Here's how the part is built. I have some questions about the finished solid (model axes, mm). Face numbers are marked on the shaded views. A direction names the side the tool comes from. Round coordinates to 2 decimals unless told otherwise and drop trailing zeros. Loops run counter-clockwise (first coordinate to the right, second up) from the corner with the lowest first, then second, coordinate; pieces in that order, holes last. Notation, with made-up numbers: M 12.25,30.25 L 30.25,30.25 A27 cw 30.25,52.25 Z; hole C -4,69 d9. An arc over 180 degrees is marked long. Answer as a JSON object with one key per item and string values.
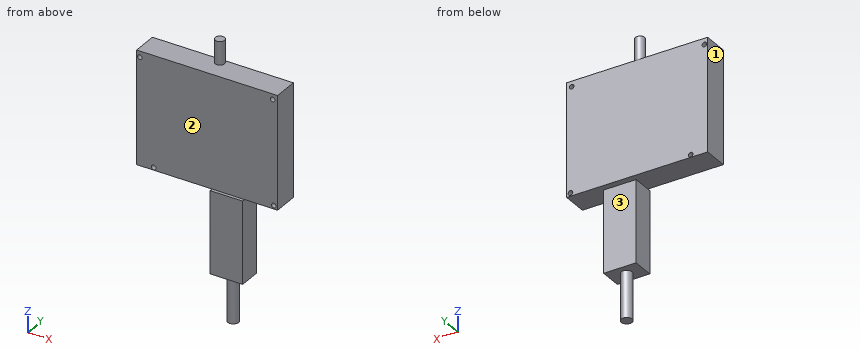
from build123d import *

# Parameters (mm, degrees)
SKETCH1_W                = 91.1
SKETCH1_H                = 73
SKETCH1_R                = 1.5
BOSS_EXTRUDE1_DEPTH      = 16.1
SKETCH2_R                = 3
BOSS_EXTRUDE2_DEPTH      = 15
BOSS_EXTRUDE3_DEPTH      = 12
BOSS_EXTRUDE3_DEPTH_BACK = 2
SKETCH3_W                = 21
SKETCH3_H                = 53
SKETCH4_R                = 3.5
BOSS_EXTRUDE4_DEPTH      = 30


with BuildPart() as part:
    # Sketch1 → Boss-Extrude1 (new body)
    with BuildSketch(Plane(origin=(0, 0, 0), x_dir=(1, 0, 0), z_dir=(0, 1, 0))):
        Rectangle(SKETCH1_W, SKETCH1_H)
        with Locations(Location((-34.59, 34.8, 0), (0, 0, 270))):
            Circle(SKETCH1_R, mode=Mode.SUBTRACT)
        with Locations(Location((43.1, 34.36, 0), (0, 0, 270))):
            Circle(SKETCH1_R, mode=Mode.SUBTRACT)
        with Locations(Location((42.3, -32.93, 0), (0, 0, 270))):
            Circle(SKETCH1_R, mode=Mode.SUBTRACT)
        with Locations(Location((-43.5, -32.58, 0), (0, 0, 270))):
            Circle(SKETCH1_R, mode=Mode.SUBTRACT)
    extrude(amount=BOSS_EXTRUDE1_DEPTH)

    # Sketch2 → Boss-Extrude2 (add)
    with BuildSketch(Plane.XY.offset(36.5)):
        with Locations(Location((0, 13.1, 0), (0, 0, 90))):
            Circle(SKETCH2_R)
    extrude(amount=BOSS_EXTRUDE2_DEPTH)

    # Sketch3 → Boss-Extrude3 (add, two sides: drawn at the far end of the back side and taken through both)
    with BuildSketch(Plane(origin=(0, 0, 0), x_dir=(1, 0, 0), z_dir=(0, 1, 0)).offset(-BOSS_EXTRUDE3_DEPTH_BACK)):
        with Locations((13.75, 63)):
            Rectangle(SKETCH3_W, SKETCH3_H)
    extrude(amount=BOSS_EXTRUDE3_DEPTH + BOSS_EXTRUDE3_DEPTH_BACK)

    # Sketch4 → Boss-Extrude4 (add)
    with BuildSketch(Plane(origin=(0, 0, -89.5), x_dir=(-1, 0, 0), z_dir=(0, 0, -1))):
        with Locations((-13.75, 5)):
            Circle(SKETCH4_R)
    extrude(amount=BOSS_EXTRUDE4_DEPTH)


solid = part.part
Item 1: For P1, Ø8, axis at x = 14.5, y = 10, coming from the +Z side; P2, Ø4, axis at y = 2.5, z = -50.5, coming from the +X side; P3, Ø1.5, axis at y = 7, z = -98.5, coming from the -X side, each with a flat end and sliding along its axis, tell me the tip position at first contact or that it passes through.
Solution:
{"P1": "stops at z = 36.5", "P2": "stops at x = 24.25", "P3": "stops at x = 10.48"}
Item 2: For the marked faces 1, 2 and 3, which set-ups out of +Z, -Z, +X, -X, +Y, -Y let a thin tool reach every point of the face, with its end or its side?
Solution:
{"face 1": "+Z, -Z, -X, +Y, -Y", "face 2": "+Z, +X, -X, -Y", "face 3": "-Z, +X, -X, +Y"}
Item 3: I want a section at C-C on x = 34. List the corners of the cut face in (y, z) for me.
Solution:
{"outline": "M 0,-36.5 L 16.1,-36.5 L 16.1,36.5 L 0,36.5 Z"}
Item 4: I want a section at B-B on x = 13.75. List the corners of the cut face in (y, z) for me, plus the area to 3 significant figures.
Solution:
{"outline": "M -2,-89.5 L 1.5,-89.5 L 1.5,-119.5 L 8.5,-119.5 L 8.5,-89.5 L 12,-89.5 L 12,-36.5 L 16.1,-36.5 L 16.1,36.5 L 0,36.5 L 0,-36.5 L -2,-36.5 Z", "area": "2,130 mm2"}
Item 5: If I drill on L1, parallel to X at y = 12.5, z = 32.58; L2, parallel to X at y = 10.5, z = -73; L3, parallel to Y at x = -25, z = 16.5, over which ranges is the centre line in solid material (lowest first)? Write a range as from..to.
Solution:
{"L1": "x = -45.55..-45, -42..40.84, 43.76..45.55", "L2": "x = 3.25..24.25", "L3": "y = 0..16.1"}
Item 6: I want a section at A-A on y = 5. List the corners of the cut face in (x, z) for me.
Solution:
{"outline": "M -45.55,-36.5 L 3.25,-36.5 L 3.25,-89.5 L 10.25,-89.5 L 10.25,-119.5 L 17.25,-119.5 L 17.25,-89.5 L 24.25,-89.5 L 24.25,-36.5 L 45.55,-36.5 L 45.55,36.5 L -45.55,36.5 Z; hole C -43.5,32.58 d3; hole C -34.59,-34.8 d3; hole C 42.3,32.93 d3; hole C 43.1,-34.36 d3"}
